Source: CAD feature listing. Evaluate the final solid. Frame: model axes, mm. A direction names the side the tool comes from. Give positions to 0.01 mm unless a question says otherwise; leave off trailing zeros. Order: outer loops, then holes, each group sorted by start corner. A loop starts at its lowest first (then second) coordinate and runs counter-clockwise, first axis right, second up. Notation, with made-up numbers: M -36.75,15 L -26.75,15 A22 cw -26.75,29 Z; hole C 26,40.25 d3. An arc over 180 degrees is marked long. Return JSON: item names as keys, results as strings.
from build123d import *

# Parameters (mm, degrees)
F0_R     = 13.46
F1_DEPTH = 43.5
F2_T     = -2
F3_W     = 6
F3_H     = 30
F4_DEPTH = 4
F5_R     = 1.35
F6_DEPTH = 43.501
F7_R     = 2.35
F7_R_2   = 1.35
F8_DEPTH = 1
F9_R     = 0.5


with BuildPart() as f1:
    # F0 (on Top) → F1 (new body)
    with BuildSketch(Plane.XY):
        Circle(F0_R)
    extrude(amount=F1_DEPTH)

    # F2
    f2_openings = [f1.faces().sort_by_distance(p)[0] for p in [
        (0, 0, 43.5),
    ]]
    offset(amount=F2_T, openings=f2_openings)

    # F3 (on face) → F4 (cut)
    with BuildSketch(Plane.XY.offset(43.5)):
        Rectangle(F3_W, F3_H)
    extrude(amount=-F4_DEPTH, mode=Mode.SUBTRACT)

    # F5 (on face) → F6 (cut, through all)
    with BuildSketch(Plane(origin=(0, 0, 0), x_dir=(1, 0, 0), z_dir=(0, 0, -1))):
        Circle(F5_R)
    extrude(amount=-F6_DEPTH, mode=Mode.SUBTRACT)

    # F7 (on face) → F8 (join)
    with BuildSketch(Plane.XY.offset(2)):
        Circle(F7_R)
        Circle(F7_R_2, mode=Mode.SUBTRACT)
    extrude(amount=F8_DEPTH)

    # F9
    f9_edges = [f1.edges().sort_by_distance(p)[0] for p in [
        (-2.35, 0, 3),
    ]]
    fillet(f9_edges, radius=F9_R)


solid = f1.part
1. Section query A-A (x = 0). Return loops of the section in (y, z).
Evaluation:
{"outline": "M -13.46,0 L -1.35,0 L -1.35,3 L -1.85,3 A0.5 ccw -2.35,2.5 L -2.35,2 L -11.46,2 L -11.46,39.5 L -13.46,39.5 Z; M 1.35,0 L 13.46,0 L 13.46,39.5 L 11.46,39.5 L 11.46,2 L 2.35,2 L 2.35,2.5 A0.5 ccw 1.85,3 L 1.35,3 Z"}
2. Section query B-B (y = 0). Return loops of the section in (x, z).
Evaluation:
{"outline": "M -13.46,0 L -1.35,0 L -1.35,3 L -1.85,3 A0.5 ccw -2.35,2.5 L -2.35,2 L -11.46,2 L -11.46,43.5 L -13.46,43.5 Z; M 1.35,0 L 13.46,0 L 13.46,43.5 L 11.46,43.5 L 11.46,2 L 2.35,2 L 2.35,2.5 A0.5 ccw 1.85,3 L 1.35,3 Z"}
3. Set-up query: faces 4 (the face through (10.93, 3.44, 22.46)), 5 (the face through (-12, -1, 43.5)), 6 (the face through (3, 12, 42)). Return all of +Z, -Z, +X, -X, +Y, -Y with unobstructed straight access to the full face (end or side cutting, diameter ignored); none if empty.
Evaluation:
{"face 4": "+Z", "face 5": "+Z, +X, -X, +Y, -Y", "face 6": "+Z, +Y, -Y"}
4. Draft query along Y for faces 1 (the face through (12.43, -5.16, 21.45)), 2 (the face through (-0.29, -1.32, 1.48)), 3 (the face through (-3, 12, 42)). Return one class per face: pulls with the +Y half, pulls with the -Y half, needs draft (parallel to the pull), parting line crosses it, or undercut.
Evaluation:
{"face 1": "parting line crosses it", "face 2": "undercut", "face 3": "needs draft"}
5. Section query C-C (z = 21). Return loops of the section in (x, y).
Evaluation:
{"outline": "C 0,0 d26.92; hole C 0,0 d22.92"}
6. Section query D-D (x = 9). Return loops of the section in (y, z).
Evaluation:
{"outline": "M -10.01,0 L 10.01,0 L 10.01,43.5 L 7.09,43.5 L 7.09,2 L -7.09,2 L -7.09,43.5 L -10.01,43.5 Z"}
7. First-contact query: pin 1 (2 mm diameter, centred on y = -10, z = 12, fed in from +X); pin 2 (1.9 mm diameter, centred on x = 0.5, y = -12, fed in from +Z); pin 3 (2 mm diameter, centred on x = 0, y = 0, fed in from +Z); pin 4 (0.6 mm diameter, centred on y = 12, z = 41.5, fed in from -X). Flat tips, straight axial feed; report the tip coordinate or a pass-through.
Evaluation:
{"pin 1": "stops at x = 10.01", "pin 2": "stops at z = 39.5", "pin 3": "passes through", "pin 4": "stops at x = -6.65"}
8. Ray query, probe 1 along Y at (x, z) = (0, 2.3); probe 2 along X at (y, z) = (3, 20.5); probe 3 along Y at (x, z) = (0, 1.75). Return the intervals inside material, ascending.
Evaluation:
{"probe 1": "y = -13.46 to -11.46, -2.35 to -1.35, 1.35 to 2.35, 11.46 to 13.46", "probe 2": "x = -13.12 to -11.06, 11.06 to 13.12", "probe 3": "y = -13.46 to -1.35, 1.35 to 13.46"}
